from build123d import *

# Parameters (mm, degrees)
F0_R      = 50
F1_DEPTH  = 15
F2_W      = 45
F2_H      = 7.5
F2_W_2    = 7.5
F2_H_2    = 45
F3_DEPTH  = 15
F5_DEPTH  = 150
F6_W      = 45
F6_H      = 10
F7_DEPTH  = 10
F8_W      = 45
F8_H      = 10
F9_DEPTH  = 10
F10_W     = 45
F10_H     = 10
F11_DEPTH = 10
F12_W     = 45
F12_H     = 10
F13_DEPTH = 10
F14_R     = 5


with BuildPart() as f1:
    # F0 (on Top) → F1 (new body)
    with BuildSketch(Plane.XY):
        Circle(F0_R)
    extrude(amount=F1_DEPTH)

    # F2 (on face) → F3 (join)
    with BuildSketch(Plane(origin=(0, 0, 0), x_dir=(1, 0, 0), z_dir=(0, 0, -1))):
        with Locations((0, 28.75)):
            Rectangle(F2_W, F2_H)
        with Locations((-28.75, 0)):
            Rectangle(F2_W_2, F2_H_2)
        with Locations((28.75, 0)):
            Rectangle(F2_W_2, F2_H_2)
        with Locations((0, -28.75)):
            Rectangle(F2_W, F2_H)
    extrude(amount=F3_DEPTH)

    # F4 (on face) → F5 (join)
    with BuildSketch(Plane(origin=(0, 0, 0), x_dir=(1, 0, 0), z_dir=(0, 0, -1))):
        Polygon((-25, -22.5), (-32.5, -22.5), (-32.5, -32.5), (-22.5, -32.5), (-22.5, -25), (-22.5, -22.5), align=None)
        Polygon((-22.5, 32.5), (-32.5, 32.5), (-32.5, 22.5), (-25, 22.5), (-22.5, 22.5), (-22.5, 25), align=None)
        Polygon((32.5, 32.5), (22.5, 32.5), (22.5, 25), (22.5, 22.5), (25, 22.5), (32.5, 22.5), align=None)
        Polygon((32.5, -32.5), (32.5, -22.5), (25, -22.5), (22.5, -22.5), (22.5, -25), (22.5, -32.5), align=None)
    extrude(amount=F5_DEPTH)

    # F6 (on face) → F7 (join)
    with BuildSketch(Plane.XZ.offset(32.5)):
        with Locations((0, -105)):
            Rectangle(F6_W, F6_H)
    extrude(amount=-F7_DEPTH)

    # F8 (on face) → F9 (join)
    with BuildSketch(Plane(origin=(0, 32.5, 0), x_dir=(-1, 0, 0), z_dir=(0, 1, 0))):
        with Locations((0, -105)):
            Rectangle(F8_W, F8_H)
    extrude(amount=-F9_DEPTH)

    # F10 (on face) → F11 (join)
    with BuildSketch(Plane(origin=(-32.5, 0, 0), x_dir=(0, -1, 0), z_dir=(-1, 0, 0))):
        with Locations((0, -113)):
            Rectangle(F10_W, F10_H)
    extrude(amount=-F11_DEPTH)

    # F12 (on face) → F13 (join)
    with BuildSketch(Plane.YZ.offset(32.5)):
        with Locations((0, -113)):
            Rectangle(F12_W, F12_H)
    extrude(amount=-F13_DEPTH)

    # F14
    f14_edges = [f1.edges().sort_by_distance(p)[0] for p in [
        (-50, 0, 15),
    ]]
    fillet(f14_edges, radius=F14_R)


solid = f1.part
Here's how the part is built. I have some questions about the finished solid (model axes, mm). A direction names the side the tool comes from. Give positions to 0.01 mm unless a question says otherwise; leave off trailing zeros. Loops run counter-clockwise (first coordinate to the right, second up) from the corner with the lowest first, then second, coordinate; pieces in that order, holes last. Notation, with made-up numbers: (-3.75, 32.25) -> (20.25, 32.25) arc R16 ccw to (20.25, 61.25) -> close; hole circle Ø5 at (-37, 50.5). An arc over 180 degrees is marked (long way). One line per item, written item: value.
Q1. Suppose I cut it at C-C on y = 0. Please give me the cut outline in (x, z).
Answers follow:
outline: (-50, 0) -> (-32.5, 0) -> (-32.5, -15) -> (-25, -15) -> (-25, 0) -> (25, 0) -> (25, -15) -> (32.5, -15) -> (32.5, 0) -> (50, 0) -> (50, 10) arc R5 ccw to (45, 15) -> (-45, 15) arc R5 ccw to (-50, 10) -> close; (-32.5, -118) -> (-22.5, -118) -> (-22.5, -108) -> (-32.5, -108) -> close; (22.5, -118) -> (32.5, -118) -> (32.5, -108) -> (22.5, -108) -> close
Q2. On a 3-axis mill with a long thin cutter (end or side, diameter ignored), from which of +Z, -Z, +X, -X, +Y, -Y can I reach the whole of each face in a straight line? I mean faces 4 (the face through (0, 28, -100)), 5 (the face through (28, 0, -108)), 6 (the face through (-28, 0, -118)), 7 (the face through (32.5, 24, -64)), 8 (the face through (0, -25, -7)). Say none if no direction works.
Answers follow:
face 4: +Y, -Y
face 5: +X, -X
face 6: -Z, +X, -X
face 7: -Z, +X, +Y, -Y
face 8: none
Q3. We'd pull the mould along Y, two halves only. Please class faces 1 (the face through (25, 0, -7)), 2 (the face through (47.69, 15.02, 4.93)), 3 (the face through (0, -29, -15)): pulls with the +Y half, pulls with the -Y half, needs draft (parallel to the pull), parting line crosses it, or undercut.
Answers follow:
face 1: undercut
face 2: parting line crosses it
face 3: needs draft
Q4. Suppose I cut it at B-B on x = 0. Please give me the cut outline in (y, z).
Answers follow:
outline: (-50, 0) -> (-32.5, 0) -> (-32.5, -15) -> (-25, -15) -> (-25, 0) -> (25, 0) -> (25, -15) -> (32.5, -15) -> (32.5, 0) -> (50, 0) -> (50, 10) arc R5 ccw to (45, 15) -> (-45, 15) arc R5 ccw to (-50, 10) -> close; (-32.5, -110) -> (-22.5, -110) -> (-22.5, -100) -> (-32.5, -100) -> close; (22.5, -110) -> (32.5, -110) -> (32.5, -100) -> (22.5, -100) -> close
Q5. If I drill on line 1 along Y through (x, z) = (-30, -100); line 2 along Z through (x, y) = (-23.5, -7), over which ranges is the centre line in solid material (lowest first)?
Answers follow:
line 1: -32.5 to -22.5, 22.5 to 32.5
line 2: -118 to -108, 0 to 15
Q6. Suppose I cut it at A-A on z = -115. Please give me the cut outline in (x, y), then the cut area to 3 significant figures.
Answers follow:
outline: (-32.5, -32.5) -> (-22.5, -32.5) -> (-22.5, 32.5) -> (-32.5, 32.5) -> close; (22.5, -32.5) -> (32.5, -32.5) -> (32.5, 32.5) -> (22.5, 32.5) -> close
area: 1,300 mm^2
Q7. Suppose I cut it at D-D on z = -42.5. Please give me the cut outline in (x, y).
Answers follow:
outline: (-32.5, -32.5) -> (-22.5, -32.5) -> (-22.5, -22.5) -> (-32.5, -22.5) -> close; (-32.5, 22.5) -> (-22.5, 22.5) -> (-22.5, 32.5) -> (-32.5, 32.5) -> close; (22.5, -32.5) -> (32.5, -32.5) -> (32.5, -22.5) -> (22.5, -22.5) -> close; (22.5, 22.5) -> (32.5, 22.5) -> (32.5, 32.5) -> (22.5, 32.5) -> close
Q8. I'm going to push flat-ended pins straight in: pin 1 Ø11 at (x, y) = (25, 8) entering from -Z; pin 2 Ø11 at (x, y) = (0.5, -27) entering from -Z; pin 3 Ø4 at (x, z) = (-27.5, -13) entering from +Y. Where does each tip first touch, or does it pass through?
Answers follow:
pin 1: z = -118
pin 2: z = -110
pin 3: y = 32.5
